Can you work these out from the model? Positions are in its coordinate system, mm. Face numbers are marked on the shaded views. A direction names the side the tool comes from. Give positions to 0.01 mm unless a question says otherwise; leave off trailing zeros. Order: outer loops, then holes, each group sorted by start corner. A loop starts at its lowest first (then second) coordinate and runs counter-clockwise, first axis right, second up. Notation, with made-up numbers: (73.5, 36) - (95.5, 36) arc R28 ccw to (95.5, 59) - close; hole circle Ø1 at (85.25, 72.25). An arc over 180 degrees is marked (long way). Use one line per item in the form item = value. Start each with the question number.
1) Suppose I cut it at D-D, the plane y = 0.5. Write out the boundary of the cut face in (x, z), and give its area (3 significant figures).
2) Suppose I cut it at A-A, the plane z = 0. Write out the boundary of the cut face in (x, y) (3 decimals).
3) Suppose I cut it at B-B, the plane y = 3.75. Write out the boundary of the cut face in (x, z).
4) We'd pull the mould along X, two halves only. Please class the marked faces 4, 5 and 6: released by +X, released by -X, zero draft, split by the parting line, or undercut.
5) Which directions (+Z, -Z, +X, -X, +Y, -Y) give clear straight access to the entire face, cutting with the end or side of a thin tool? Please do the marked faces 1, 2 and 3.
6) Suppose I cut it at C-C, the plane x = 0. Write out the boundary of the cut face in (y, z) (3 decimals).
7) Please list where these lines run through material, in increasing order: probe 1 along X at (y, z) = (5.6, 0); probe 2 along Y at (x, z) = (9.25, -4.5) (3 decimals); probe 3 along Z at (x, y) = (-2, 5).
8) For pin 1 (3 mm diameter, centred on x = 6, y = -2, fed in from -Z); pin 2 (1 mm diameter, centred on x = -2, z = 1, fed in from +Y) (3 decimals); pin 3 (1.5 mm diameter, centred on x = 6, y = 0, fed in from +Z); pin 4 (10 mm diameter, centred on y = -5.5, z = -2.5, fed in from +X), each with a flat end and sliding along its axis, tell me the tip position at first contact or that it passes through.
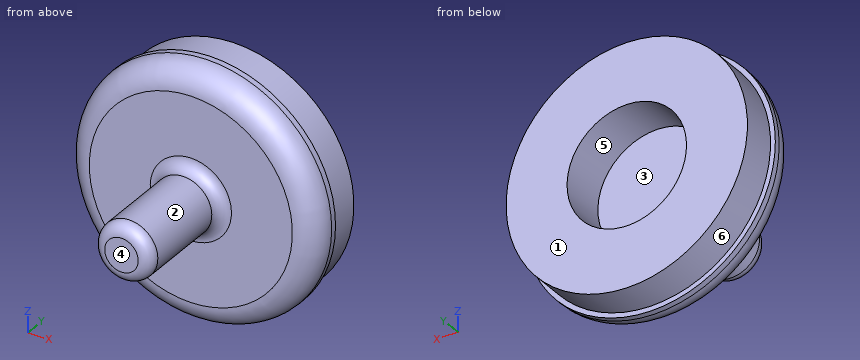
```python
from build123d import *

# Parameters (mm, degrees)
SKETCH1_R           = 13.335
BOSS_EXTRUDE1_DEPTH = 3.175
SKETCH2_R           = 12.827
BOSS_EXTRUDE2_DEPTH = 3.81
SKETCH3_R           = 6.35
CUT_EXTRUDE2_DEPTH  = 5.08
FILLET1_R           = 2.54
SKETCH5_R           = 3.048
BOSS_EXTRUDE3_DEPTH = 11.43
FILLET2_R           = 1.27
FILLET3_R           = 1.27


with BuildPart() as part:
    # Sketch1 → Boss-Extrude1 (new body)
    with BuildSketch(Plane(origin=(0, 0, 0), x_dir=(1, 0, 0), z_dir=(0, 1, 0))):
        with Locations(Location((0, 0, 0), (0, 0, 270))):
            Circle(SKETCH1_R)
    extrude(amount=BOSS_EXTRUDE1_DEPTH)

    # Sketch2 → Boss-Extrude2 (add)
    with BuildSketch(Plane(origin=(0, 3.175, 0), x_dir=(1, 0, 0), z_dir=(0, 1, 0))):
        with Locations(Location((0, 0, 0), (0, 0, 90))):
            Circle(SKETCH2_R)
    extrude(amount=BOSS_EXTRUDE2_DEPTH)

    # Sketch3 → Cut-Extrude2 (cut)
    with BuildSketch(Plane(origin=(0, 6.985, 0), x_dir=(1, 0, 0), z_dir=(0, 1, 0))):
        with Locations(Location((0, 0, 0), (0, 0, 270))):
            Circle(SKETCH3_R)
    extrude(amount=-CUT_EXTRUDE2_DEPTH, mode=Mode.SUBTRACT)

    # Fillet1
    fillet1_edges = [part.edges().sort_by_distance(p)[0] for p in [
        (0, 0, -13.335),
    ]]
    fillet(fillet1_edges, radius=FILLET1_R)

    # Sketch5 → Boss-Extrude3 (add)
    with BuildSketch(Plane.XZ):
        with Locations(Location((0, 0, 0), (0, 0, 90))):
            Circle(SKETCH5_R)
    extrude(amount=BOSS_EXTRUDE3_DEPTH)

    # Fillet2
    fillet2_edges = [part.edges().sort_by_distance(p)[0] for p in [
        (0, -11.43, -3.048),
    ]]
    fillet(fillet2_edges, radius=FILLET2_R)

    # Fillet3
    fillet3_edges = [part.edges().sort_by_distance(p)[0] for p in [
        (0, 0, -3.048),
    ]]
    fillet(fillet3_edges, radius=FILLET3_R)


solid = part.part
```
Result sheet:
q1.outline = circle Ø24.62 at (0, 0)
q1.area = 476 mm²
q2.outline = (-13.335, 2.54) arc R2.54 ccw to (-10.795, 0) - (-4.318, 0) arc R1.27 cw to (-3.048, -1.27) - (-3.048, -10.16) arc R1.27 ccw to (-1.778, -11.43) - (1.778, -11.43) arc R1.27 ccw to (3.048, -10.16) - (3.048, -1.27) arc R1.27 cw to (4.318, 0) - (10.795, 0) arc R2.54 ccw to (13.335, 2.54) - (13.335, 3.175) - (12.827, 3.175) - (12.827, 6.985) - (6.35, 6.985) - (6.35, 1.905) - (-6.35, 1.905) - (-6.35, 6.985) - (-12.827, 6.985) - (-12.827, 3.175) - (-13.335, 3.175) - close
q3.outline = circle Ø25.65 at (0, 0); hole circle Ø12.7 at (0, 0)
q4.face_4 = zero draft
q4.face_5 = undercut
q4.face_6 = split by the parting line
q5.face_1 = +Z, -Z, +X, -X, +Y
q5.face_2 = -Y
q5.face_3 = +Y
q6.outline = (-11.43, -1.778) arc R1.27 ccw to (-10.16, -3.048) - (-1.27, -3.048) arc R1.27 cw to (0, -4.318) - (0, -10.795) arc R2.54 ccw to (2.54, -13.335) - (3.175, -13.335) - (3.175, -12.827) - (6.985, -12.827) - (6.985, -6.35) - (1.905, -6.35) - (1.905, 6.35) - (6.985, 6.35) - (6.985, 12.827) - (3.175, 12.827) - (3.175, 13.335) - (2.54, 13.335) arc R2.54 ccw to (0, 10.795) - (0, 4.318) arc R1.27 cw to (-1.27, 3.048) - (-10.16, 3.048) arc R1.27 ccw to (-11.43, 1.778) - close
q7.probe_1 = -12.83 to -6.35, 6.35 to 12.83
q7.probe_2 = 0 to 6.985
q7.probe_3 = -12.67 to -6.03, 6.03 to 12.67
q8.pin_1 = through
q8.pin_2 = 1.905
q8.pin_3 = 11.16
q8.pin_4 = 3.06
